Source: CAD feature listing. Evaluate the final solid. Frame: model axes, mm. Face numbers are marked on the shaded views. A direction names the side the tool comes from. Give positions to 0.01 mm unless a question says otherwise; leave off trailing zeros. Loops run counter-clockwise (first coordinate to the right, second up) from the corner with the lowest first, then second, coordinate; pieces in that order, holes last. Notation, with made-up numbers: (80, 42.25) - (122, 42.25) arc R16 cw to (122, 58.25) - close; hole circle Ø3 at (58.5, -3.75). An arc over 180 degrees is marked (long way). Put each result on its own line as item: value.
```python
from build123d import *

# Parameters (mm, degrees)
SKETCH1_R           = 5
BOSS_EXTRUDE1_DEPTH = 5
FILLET1_R           = 1
SKETCH2_R           = 2
CUT_EXTRUDE1_DEPTH  = 5
SKETCH4_R           = 1
CUT_EXTRUDE2_DEPTH  = 10


with BuildPart() as part:
    # Sketch1 → Boss-Extrude1 (new body)
    with BuildSketch(Plane.XY):
        Circle(SKETCH1_R)
    extrude(amount=BOSS_EXTRUDE1_DEPTH)

    # Fillet1
    fillet1_edges = [part.edges().sort_by_distance(p)[0] for p in [
        (-5, 0, 0),
        (-5, 0, 5),
    ]]
    fillet(fillet1_edges, radius=FILLET1_R)

    # Sketch2 → Cut-Extrude1 (cut)
    with BuildSketch(Plane(origin=(0, 0, 0), x_dir=(-1, 0, 0), z_dir=(0, 0, -1))):
        Circle(SKETCH2_R)
    extrude(amount=-CUT_EXTRUDE1_DEPTH, mode=Mode.SUBTRACT)

    # Sketch3 → Revolve1 (revolve)
    with BuildSketch(Plane(origin=(0, 0, 0), x_dir=(1, 0, 0), z_dir=(0, 1, 0)), mode=Mode.PRIVATE) as revolve1_sk:
        Polygon((4.094510591, -1), (8, -1), (8, -0.5), (11, -1), (11, -2.5), (4.094510591, -2.5), align=None)
    revolve(revolve1_sk.sketch.rotate(Axis((5, 0, 2.5), (1, 0, 0)), 180), axis=Axis((5, 0, 2.5), (1, 0, 0)))

    # Sketch4 → Cut-Extrude2 (cut)
    with BuildSketch(Plane(origin=(11, 0, 0), x_dir=(0, 0, -1), z_dir=(1, 0, 0))):
        with Locations((-2.5, 0)):
            Circle(SKETCH4_R)
    extrude(amount=-CUT_EXTRUDE2_DEPTH, mode=Mode.SUBTRACT)


solid = part.part
```
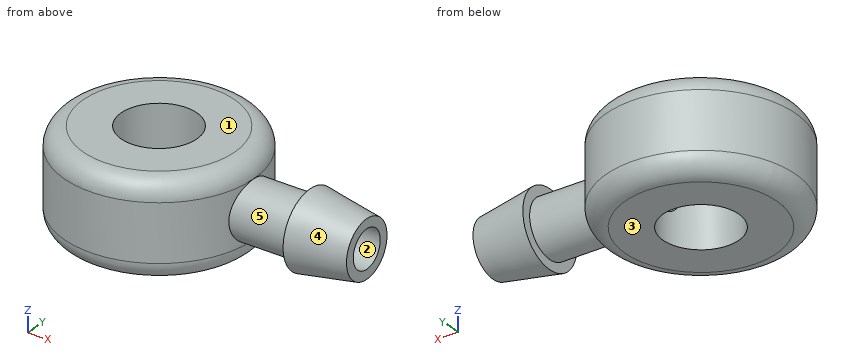
1) Section query C-C, the plane y = -0.75. State how many separate pieces and enclosed holes the cut face has, plus the area to 3 significant figures.
Check result:
separate pieces: 3
enclosed holes: 0
area: 35.3 mm²
2) Mould query, pull axis Z, two halves, no side actions, for the marked faces 1, 2 and 3. Classes: pulls with the +Z half, pulls with the -Z half, needs draft (parallel to the pull), parting line crosses it, or undercut.
Check result:
face 1: pulls with the +Z half
face 2: undercut
face 3: pulls with the -Z half
3) Material intervals for line 1 along Y through (x, z) = (7, 2.5); line 2 along Y through (x, z) = (0, 1.3); line 3 along X through (y, z) = (-1.5, 0.8), sorted ascending. Write a range as [from, to].
Check result:
line 1: [-1.5, -1], [1, 1.5]
line 2: [-5, -2], [2, 5]
line 3: [-4.75, -1.32], [1.32, 4.75]
4) Section query B-B, the plane z = 2.5. Output: boundary loops of the cut face in (x, y), plus the area to 3 significant figures.
Check result:
outline: (1.73, -1) arc R2 cw (long way) to (1.73, 1) - (11, 1) - (11, 1.5) - (8, 2) - (8, 1.5) - (4.77, 1.5) arc R5 ccw (long way) to (4.77, -1.5) - (8, -1.5) - (8, -2) - (11, -1.5) - (11, -1) - close
area: 67.5 mm²
5) Access query for the marked faces 4 and 5. Directions: +Z, -Z, +X, -X, +Y, -Y. A direction counts if a zero-diameter tool reaches every point of the face in a straight line with its end or side. Return the directions, or none.
Check result:
face 4: +X
face 5: none
6) Section query A-A, the plane x = 0. Output: boundary loops of the cut face in (y, z), plus the area to 3 significant figures.
Check result:
outline: (-5, 1) arc R1 ccw to (-4, 0) - (-2, 0) - (-2, 5) - (-4, 5) arc R1 ccw to (-5, 4) - close; (2, 0) - (4, 0) arc R1 ccw to (5, 1) - (5, 4) arc R1 ccw to (4, 5) - (2, 5) - close
area: 29.1 mm²
7) Pin query (flat end, axial travel): P1, Ø3, axis at x = 7, z = 2.5, coming from the -Y side; P2, Ø1, axis at x = 4, z = 4, coming from the +Y side; P3, Ø1, axis at x = -3, z = 4, coming from the +Y side. Return the tip coordinate at first contact, or that it passes through.
Check result:
P1: y = -2
P2: y = 3.57
P3: y = 4.33
